```python
from build123d import *

# Parameters (mm, degrees)
F0_R     = 3
F0_R_2   = 2.5
F1_DEPTH = 5
F2_R     = 6
F3_DEPTH = 2.5


with BuildPart() as f1:
    # F0 (on Front) → F1 (new body)
    with BuildSketch(Plane.XZ):
        with BuildLine():
            ThreePointArc((-38.5, -33.5), (-37.035534, -37.035534), (-33.5, -38.5))
            Line((-33.5, -38.5), (33.5, -38.5))
            ThreePointArc((33.5, -38.5), (37.035534, -37.035534), (38.5, -33.5))
            Line((38.5, -33.5), (38.5, 33.5))
            ThreePointArc((38.5, 33.5), (37.035534, 37.035534), (33.5, 38.5))
            Line((33.5, 38.5), (-33.5, 38.5))
            ThreePointArc((-33.5, 38.5), (-37.035534, 37.035534), (-38.5, 33.5))
            Line((-38.5, 33.5), (-38.5, -33.5))
        make_face()
        with Locations((-14.5, -30.5)):
            Circle(F0_R, mode=Mode.SUBTRACT)
        with Locations((-10, -19.5)):
            Circle(F0_R_2, mode=Mode.SUBTRACT)
        with Locations((14.5, -30.5)):
            Circle(F0_R_2, mode=Mode.SUBTRACT)
        with Locations((10, -19.5)):
            Circle(F0_R_2, mode=Mode.SUBTRACT)
        with Locations((-10, 0)):
            Circle(F0_R_2, mode=Mode.SUBTRACT)
        with Locations((-10, 19.5)):
            Circle(F0_R_2, mode=Mode.SUBTRACT)
        with Locations((-14.5, 30.5)):
            Circle(F0_R, mode=Mode.SUBTRACT)
        with Locations((10, 0)):
            Circle(F0_R_2, mode=Mode.SUBTRACT)
        with Locations((10, 19.5)):
            Circle(F0_R_2, mode=Mode.SUBTRACT)
        with Locations((14.5, 30.5)):
            Circle(F0_R_2, mode=Mode.SUBTRACT)
    extrude(amount=F1_DEPTH)

    # F2 (on face) → F3 (cut)
    with BuildSketch(Plane.XZ.offset(5)):
        with Locations((-14.5, 30.5)):
            Circle(F2_R)
        with Locations((-14.5, -30.5)):
            Circle(F2_R)
        with Locations((14.5, 30.5)):
            Circle(F2_R)
        with Locations((14.5, -30.5)):
            Circle(F2_R)
    extrude(amount=-F3_DEPTH, mode=Mode.SUBTRACT)


solid = f1.part
```
Build history of the part. All positions in model axes, mm. A direction names the side the tool comes from. Give positions to 0.01 mm unless a question says otherwise; leave off trailing zeros. Loops run counter-clockwise (first coordinate to the right, second up) from the corner with the lowest first, then second, coordinate; pieces in that order, holes last. Notation, with made-up numbers: (43.5, -6) -> (60.5, -6) arc R22 ccw to (60.5, 16) -> close; hole circle Ø5 at (-18, -21.5). An arc over 180 degrees is marked (long way). One line per question, with ' | ' between items. Start each with the question number.
1) Cut at D-D (z = -19.5). Give the cut face in (x, y).
2) Two-plate mould, pull along Z, no slides. Class faces 1 (the flat face through (38.5, -2, 0)), 2 (the cylindrical face through (-11.731, -3.768, 25.177)), 3 (the cylindrical face through (37, -2.46, -37.07)): released by +Z, released by -Z, zero draft, split by the parting line, or undercut.
3) Pin check, flat tips, straight feed: pin 1 (11 mm diameter, centred on x = 14.5, z = 30.5, fed in from -Y); pin 2 (12 mm diameter, centred on x = 4.5, z = 19, fed in from +Y); pin 3 (3 mm diameter, centred on x = 14.5, z = 30.5, fed in from -Y). Stop position of each tip, or through.
4) 3-axis set-ups, long thin cutter, end or side, ignore diameter. For faces 4 (the cylindrical face through (-37, -2.46, 37.07)), 5 (the cylindrical face through (-11.731, -3.768, -35.823)): which of +Z, -Z, +X, -X, +Y, -Y reach the whole face in a straight line?
5) Cut at A-A (z = -30.5). Give the cut face in (x, y).
6) Cut at C-C (x = -14.5). Give the cut face in (y, z), plus the area to 3 significant figures.
7) Probe L1, parallel to X at y = -0.9, z = 30.5; L2, parallel to Z at x = 10, y = -1.3; L3, parallel to Z at x = 14.5, y = -4.2. List the from-to ranges inside material, lowest first.
8) Cut at B-B (y = -3.9). Count the separate pieces of the cut face and the enclosed holes in it, plus the area to 3 significant figures.
Return value:
1) outline: (-38.5, -5) -> (-12.5, -5) -> (-12.5, 0) -> (-38.5, 0) -> close; (-7.5, -5) -> (7.5, -5) -> (7.5, 0) -> (-7.5, 0) -> close; (12.5, -5) -> (38.5, -5) -> (38.5, 0) -> (12.5, 0) -> close
2) face 1: zero draft | face 2: undercut | face 3: released by -Z
3) pin 1: y = -2.5 | pin 2: y = 0 | pin 3: through
4) face 4: +Z, -X, +Y, -Y | face 5: -Y
5) outline: (-38.5, -5) -> (-20.5, -5) -> (-20.5, -2.5) -> (-17.5, -2.5) -> (-17.5, 0) -> (-38.5, 0) -> close; (-11.5, -2.5) -> (-8.5, -2.5) -> (-8.5, -5) -> (8.5, -5) -> (8.5, -2.5) -> (12, -2.5) -> (12, 0) -> (-11.5, 0) -> close; (17, -2.5) -> (20.5, -2.5) -> (20.5, -5) -> (38.5, -5) -> (38.5, 0) -> (17, 0) -> close
6) outline: (-5, -38.5) -> (0, -38.5) -> (0, -33.5) -> (-2.5, -33.5) -> (-2.5, -36.5) -> (-5, -36.5) -> close; (-5, -24.5) -> (-2.5, -24.5) -> (-2.5, -27.5) -> (0, -27.5) -> (0, 27.5) -> (-2.5, 27.5) -> (-2.5, 24.5) -> (-5, 24.5) -> close; (-5, 36.5) -> (-2.5, 36.5) -> (-2.5, 33.5) -> (0, 33.5) -> (0, 38.5) -> (-5, 38.5) -> close | area: 295 mm^2
7) L1: -38.5 to -17.5, -11.5 to 12, 17 to 38.5 | L2: -38.5 to -22, -17 to -2.5, 2.5 to 17, 22 to 38.5 | L3: -38.5 to -36.5, -24.5 to 24.5, 36.5 to 38.5
8) separate pieces: 1 | enclosed holes: 10 | area: 5,340 mm^2
